Geometry: final body of the model. Coordinates: model frame, mm. Give positions to 0.01 mm unless a question says otherwise; leave off trailing zeros. Write each loop counter-clockwise with the first axis right and the second up, starting at its lowest first coordinate (ties: lowest second). Pieces come first, ordered by that corner, then holes. Notation, with made-up numbers: M 77,-19.5 L 115,-19.5 A29 cw 115,1.5 Z; hole C 37,19.5 d8. An arc over 180 degrees is marked long. Answer as a JSON object with one key per item and string values.
from build123d import *

# Parameters (mm, degrees)
SKETCH010_R      = 9.5
EXTRUDE004_DEPTH = 30
ARRAY003_COUNT   = 6
SKETCH005_W      = 100
SKETCH005_H      = 15


with BuildPart() as array003:
    # Sketch010 (on Face3 of Revolve) → Extrude004 (new body)
    with BuildSketch(Plane.XY.offset(15)):
        with Locations((185, -0.1655)):
            Circle(SKETCH010_R)
    extrude(amount=-EXTRUDE004_DEPTH)

    # Array003: Array003 ×6 about axis
    array003_axis = Axis((0, 0, 590.09), (0, 0, 1))


with BuildPart() as array003_1:
    add(array003.part)
    for i in range(1, ARRAY003_COUNT):
        add(array003.part.rotate(array003_axis, i * 360 / ARRAY003_COUNT))


with BuildPart() as cut005:
    # Sketch005 → Revolve (revolve)
    with BuildSketch(Plane.XZ):
        with Locations((160, 7.5)):
            Rectangle(SKETCH005_W, SKETCH005_H)
    revolve(axis=Axis((0, 0, 0), (0, 0, 1)))

    # Cut005: cut Array003
    add(array003_1.part, mode=Mode.SUBTRACT)


solid = cut005.part
1) Contact query for flat-ended pins moving along their axis: P1, Ø22, axis at x = -185, y = 0.17, coming from the -Z side; P2, Ø6, axis at x = 21.5, z = 13, coming from the +Y side; P3, Ø1, axis at y = -22, z = 10, coming from the -X side; P4, Ø4, axis at y = 40.5, z = 11.5, coming from the -X side. Output: stop coordinate, or through.
Geometry check:
{"P1": "stops at z = 0", "P2": "stops at y = 209.18", "P3": "stops at x = -208.9", "P4": "stops at x = -206.44"}
2) Cut plane C-C on z = 3. Return loops of the section in (x, y), and give its area (3 significant figures).
Geometry check:
{"outline": "C 0,0 d420; hole C -185,0.17 d19; hole C 0,0 d220; hole C -92.64,-160.13 d19; hole C -92.36,160.3 d19; hole C 92.36,-160.3 d19; hole C 92.64,160.13 d19; hole C 185,-0.17 d19", "area": "98,800 mm2"}
3) Line query: line 1 (Y direction, x = 92, z = 6.5) (3 decimals); line 2 (Y direction, x = -2, z = 5); line 3 (X direction, y = -146, z = 13). Output: solid intervals per line, ascending. Write a range as from..to.
Geometry check:
{"line 1": "y = -188.775..-169.791, -150.804..-60.299, 60.299..150.654, 169.61..188.775", "line 2": "y = -209.99..-109.98, 109.98..209.99", "line 3": "x = -150.94..150.94"}
4) Cut plane D-D on x = -144. Return loops of the section in (y, z), and give its area (3 significant figures).
Geometry check:
{"outline": "M -152.85,0 L 152.85,0 L 152.85,15 L -152.85,15 Z", "area": "4,590 mm2"}
5) Cut plane B-B on y = 92. Return loops of the section in (x, z) (3 decimals), and give its area (3 significant figures).
Geometry check:
{"outline": "M -188.775,0 L -60.299,0 L -60.299,15 L -188.775,15 Z; M 60.299,0 L 188.775,0 L 188.775,15 L 60.299,15 Z", "area": "3,850 mm2"}
6) Pull-direction query (X, two-part tool) for faces 1 (the flat face through (-90, -90, 15)), 2 (the cylindrical face through (93.88, 150.713, 7.605)), 3 (the cylindrical face through (200.3, 63.08, 7.6)); classes: pulls with the +X half, pulls with the -X half, needs draft (parallel to the pull), parting line crosses it, or undercut.
Geometry check:
{"face 1": "needs draft", "face 2": "undercut", "face 3": "parting line crosses it"}
7) Cut plane A-A on x = 0. Return loops of the section in (y, z), and give its area (3 significant figures).
Geometry check:
{"outline": "M -210,0 L -110,0 L -110,15 L -210,15 Z; M 110,0 L 210,0 L 210,15 L 110,15 Z", "area": "3,000 mm2"}
